Geometry check sheet. Reference: the model listing, model coordinates, mm. Face numbers are marked on the shaded views. Coordinates: 2 decimals unless noted, no trailing zeros. Loops run counter-clockwise (first coordinate to the right, second up) from the corner with the lowest first, then second, coordinate; pieces in that order, holes last. Notation, with made-up numbers: M -15,88.5 L -8,88.5 A12 ccw -8,94.5 Z; hole C 76,58.5 d10. An arc over 180 degrees is marked long. One line per question, with ' | ' between items. Start each with the question number.
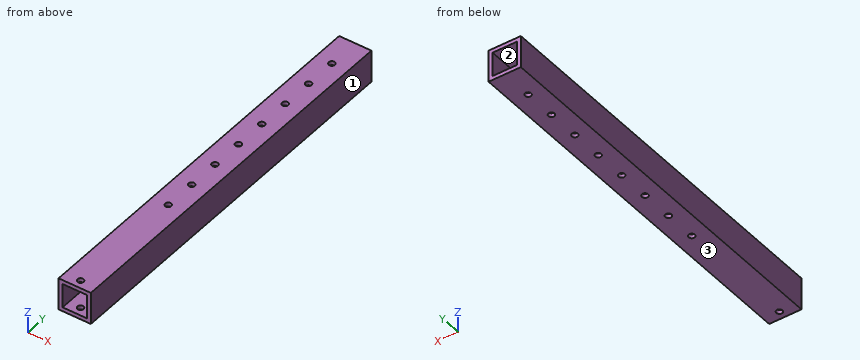
from build123d import *

# Parameters (mm, degrees)
SKETCH2_W           = 50.8
SKETCH2_H           = 50.8
SKETCH2_W_2         = 38.1
SKETCH2_H_2         = 38.1
BOSS_EXTRUDE1_DEPTH = 609.6
SKETCH3_R           = 4.826
CUT_EXTRUDE1_DEPTH  = 609.6


with BuildPart() as part:
    # Sketch2 → Boss-Extrude1 (new body)
    with BuildSketch(Plane(origin=(0, 0, 0), x_dir=(1, 0, 0), z_dir=(0, 1, 0))):
        Rectangle(SKETCH2_W, SKETCH2_H)
        Rectangle(SKETCH2_W_2, SKETCH2_H_2, mode=Mode.SUBTRACT)
    extrude(amount=BOSS_EXTRUDE1_DEPTH)

    # Sketch3 → Cut-Extrude1 (cut)
    with BuildSketch(Plane.XY.offset(25.4)):
        with Locations((0, 12.7)):
            Circle(SKETCH3_R)
        with Locations((0, 558.8)):
            Circle(SKETCH3_R)
        with Locations((0, 508)):
            Circle(SKETCH3_R)
        with Locations((0, 457.2)):
            Circle(SKETCH3_R)
        with Locations((0, 406.4)):
            Circle(SKETCH3_R)
        with Locations((0, 355.6)):
            Circle(SKETCH3_R)
        with Locations((0, 304.8)):
            Circle(SKETCH3_R)
        with Locations((0, 254)):
            Circle(SKETCH3_R)
        with Locations((0, 203.2)):
            Circle(SKETCH3_R)
    extrude(amount=-CUT_EXTRUDE1_DEPTH, mode=Mode.SUBTRACT)


solid = part.part
1. Thickness scan on line 1 (X direction, y = 52.5, z = -19); line 2 (X direction, y = 558.8, z = -21). Record the ranges inside material, lowest first.
2. Draft check along X on the marked faces 1, 2 and 3. Enter one of: +X half, -X half, draft (parallel to the pull), parting line (faces both ways), or undercut.
3. Sectioned sample at A-A (z = 7.5). Record the cut outline in (x, y).
4. Sectioned sample at B-B (y = 486). Record the cut outline in (x, z), and give its area (3 significant figures).
Result:
1) line 1: x = -25.4 to -19.05, 19.05 to 25.4 | line 2: x = -25.4 to -4.83, 4.83 to 25.4
2) face 1: +X half | face 2: undercut | face 3: draft
3) outline: M -25.4,0 L -19.05,0 L -19.05,609.6 L -25.4,609.6 Z; M 19.05,0 L 25.4,0 L 25.4,609.6 L 19.05,609.6 Z
4) outline: M -25.4,-25.4 L 25.4,-25.4 L 25.4,25.4 L -25.4,25.4 Z; hole M -19.05,-19.05 L 19.05,-19.05 L 19.05,19.05 L -19.05,19.05 Z | area: 1,130 mm2
